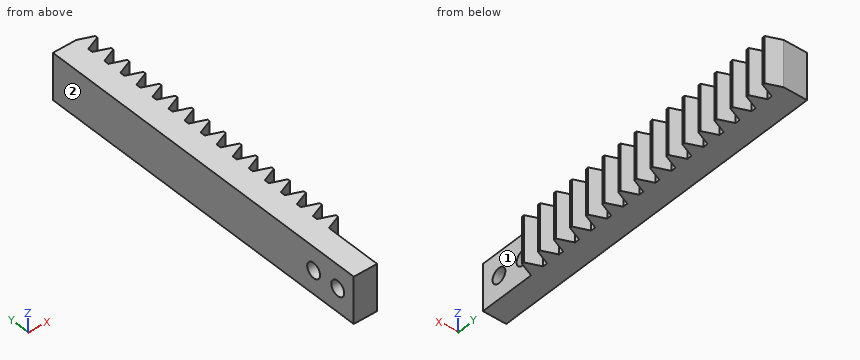
```python
from build123d import *

# Parameters (mm, degrees)
ESQUISSE1_W                = 10
ESQUISSE1_H                = 75
BOSS_EXTRU_1_DEPTH         = 5
BOSS_EXTRU_2_DEPTH         = 10
R_P_TITION_LIN_AIRE1_COUNT = 16
R_P_TITION_LIN_AIRE1_PITCH = 4
ESQUISSE3_R                = 1.6
ENL_V_MAT_EXTRU_1_DEPTH    = 10


with BuildPart() as part:
    # Esquisse1 → Boss.-Extru.1 (new body)
    with BuildSketch(Plane(origin=(0, 0, 0), x_dir=(0, 0, -1), z_dir=(1, 0, 0))):
        with Locations((5, 37.5)):
            Rectangle(ESQUISSE1_W, ESQUISSE1_H)
    extrude(amount=-BOSS_EXTRU_1_DEPTH)

    # Esquisse2 → Boss.-Extru.2 (add)
    with BuildSketch(Plane.XY):
        Polygon((0, 75), (3, 73.75), (3, 73.25), (0, 72), align=None)
    boss_extru_2 = extrude(amount=-BOSS_EXTRU_2_DEPTH)

    # Répétition linéaire1: Boss.-Extru.2 ×16
    with Locations(*[(0, -i * R_P_TITION_LIN_AIRE1_PITCH, 0) for i in range(1, R_P_TITION_LIN_AIRE1_COUNT)]):
        add(boss_extru_2)

    # Esquisse3 → Enlèv. mat.-Extru.1 (cut)
    with BuildSketch(Plane(origin=(0, 0, 0), x_dir=(0, 0, -1), z_dir=(1, 0, 0))):
        with Locations((5, 10)):
            Circle(ESQUISSE3_R)
        with Locations((5, 4)):
            Circle(ESQUISSE3_R)
    extrude(amount=-ENL_V_MAT_EXTRU_1_DEPTH, mode=Mode.SUBTRACT)


solid = part.part
```
Verification items for the finished model (mm, model axes). Face numbers are marked on the shaded views. A direction names the side the tool comes from. Coordinates: 2 decimals unless noted, no trailing zeros. Loops run counter-clockwise (first coordinate to the right, second up) from the corner with the lowest first, then second, coordinate; pieces in that order, holes last. Notation, with made-up numbers: (-22.5, 83) -> (24.5, 83) arc R23 cw to (24.5, 92) -> close; hole circle Ø2 at (63.5, -19). An arc over 180 degrees is marked (long way). Put each result on its own line as item: value.
1. Thickness scan on line 1 (Y direction, x = -1.7, z = -5); line 2 (Y direction, x = -0.75, z = -4.25); line 3 (X direction, y = 34, z = -0.25). Record the ranges inside material, lowest first.
Result set:
line 1: y = 0 to 2.4, 5.6 to 8.4, 11.6 to 75
line 2: y = 0 to 2.59, 5.41 to 8.59, 11.41 to 75
line 3: x = -5 to 2.4
2. Section check B-B, the plane x = -2. Record the boundary of the cut face in (y, z).
Result set:
outline: (0, -10) -> (75, -10) -> (75, 0) -> (0, 0) -> close; hole circle Ø3.2 at (4, -5); hole circle Ø3.2 at (10, -5)
3. Tool access check on the marked faces 1 and 2. Record the directions out of +Z, -Z, +X, -X, +Y, -Y that give a thin tool (end or side, any length) a straight path to the whole face; none if there is none.
Result set:
face 1: +Z, -Z, +X, -Y
face 2: +Z, -Z, -X, +Y, -Y
4. Gauge pin test, flat ends, axial feed: P1, Ø0.5, axis at y = 63.5, z = -6, coming from the +X side; P2, Ø1.1, axis at y = 51.5, z = -7, coming from the +X side; P3, Ø6, axis at y = 11, z = -4.5, coming from the +X side. Record the tip position at first contact, or that the pin passes through.
Result set:
P1: stops at x = 0
P2: stops at x = 0.12
P3: stops at x = 3
5. Section check A-A, the plane y = 10. Record the boundary of the cut face in (x, z), then the cut area to 3 significant figures.
Result set:
outline: (-5, -10) -> (0, -10) -> (0, -6.6) -> (-5, -6.6) -> close; (-5, -3.4) -> (0, -3.4) -> (0, 0) -> (-5, 0) -> close
area: 34.0 mm^2
6. Section check C-C, the plane z = -5. Give the number of separate pieces and of enclosed holes in the cut face, then the cut area to 3 significant figures.
Result set:
separate pieces: 3
enclosed holes: 0
area: 427 mm^2
